For this review, take the finished solid that the model builds, in its own axes (mm). Coordinates: 2 decimals unless noted, no trailing zeros. Write each loop counter-clockwise with the first axis right and the second up, starting at its lowest first coordinate (ties: lowest second). Pieces come first, ordered by that corner, then holes.
1) We need section C-C on x = -3.4. Write out the cut boundary in (y, z), then the cut area to 3 significant figures.
2) We need section A-A on z = 0. Write out the cut boundary in (x, y).
3) To check wall thickness, follow line 1 along X through (y, z) = (-9.5, 0); line 2 along Y through (x, z) = (-2.8, 0); line 3 along Y through (x, z) = (-0.4, -0.05). State the ranges of each line that lie inside material, in increasing order.
4) We need section B-B on y = -7.5. Write out the cut boundary in (x, z).
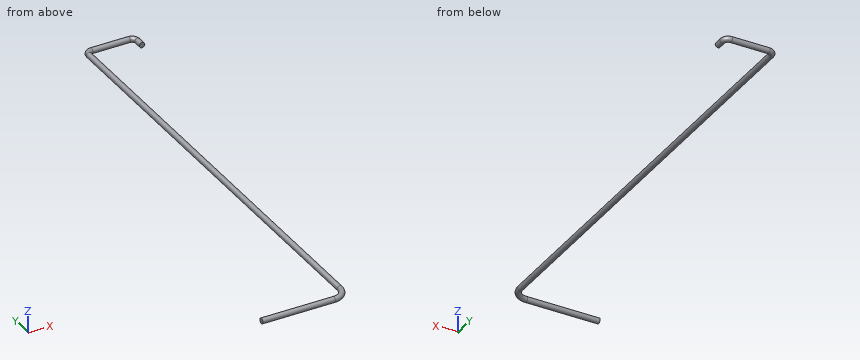
from build123d import *

# Parameters (mm, degrees)
ESQUISSE2_R = 0.1


with BuildPart() as part:
    # Balayage1: sweep along a path in Esquisse1
    with BuildLine(Plane.XY) as balayage1_path:
        Line((0, 0), (0, 0.3))
        ThreePointArc((0, 0.3), (-0.058578644, 0.441421356), (-0.2, 0.5))
        Line((-0.2, 0.5), (-1.584533741, 0.5))
        ThreePointArc((-1.584533741, 0.5), (-1.725955098, 0.441421356), (-1.784533741, 0.3))
        Line((-1.784533741, 0.3), (-1.784533741, -16.05))
        ThreePointArc((-1.784533741, -16.05), (-1.930980351, -16.403553391), (-2.284533741, -16.55))
        Line((-2.284533741, -16.55), (-4.954533741, -16.55))
    # Esquisse2 → Balayage1 (sweep)
    with BuildSketch(Plane(origin=(0, 0, 0), x_dir=(1, 0, 0), z_dir=(0, 1, 0))):
        Circle(ESQUISSE2_R)
    sweep(path=balayage1_path.line)


solid = part.part
Result:
1. outline: circle Ø0.2 at (-16.55, 0)
1. area: 0.0314 mm2
2. outline: (-4.95, -16.65) - (-2.28, -16.65) arc R0.6 ccw to (-1.68, -16.05) - (-1.68, 0.3) arc R0.1 cw to (-1.58, 0.4) - (-0.2, 0.4) arc R0.1 cw to (-0.1, 0.3) - (-0.1, 0) - (0.1, 0) - (0.1, 0.3) arc R0.3 ccw to (-0.2, 0.6) - (-1.58, 0.6) arc R0.3 ccw to (-1.88, 0.3) - (-1.88, -16.05) arc R0.4 cw to (-2.28, -16.45) - (-4.95, -16.45) - close
3. line 1: x = -1.88 to -1.68
3. line 2: y = -16.65 to -16.45
3. line 3: y = 0.41 to 0.59
4. outline: circle Ø0.2 at (-1.78, 0)
